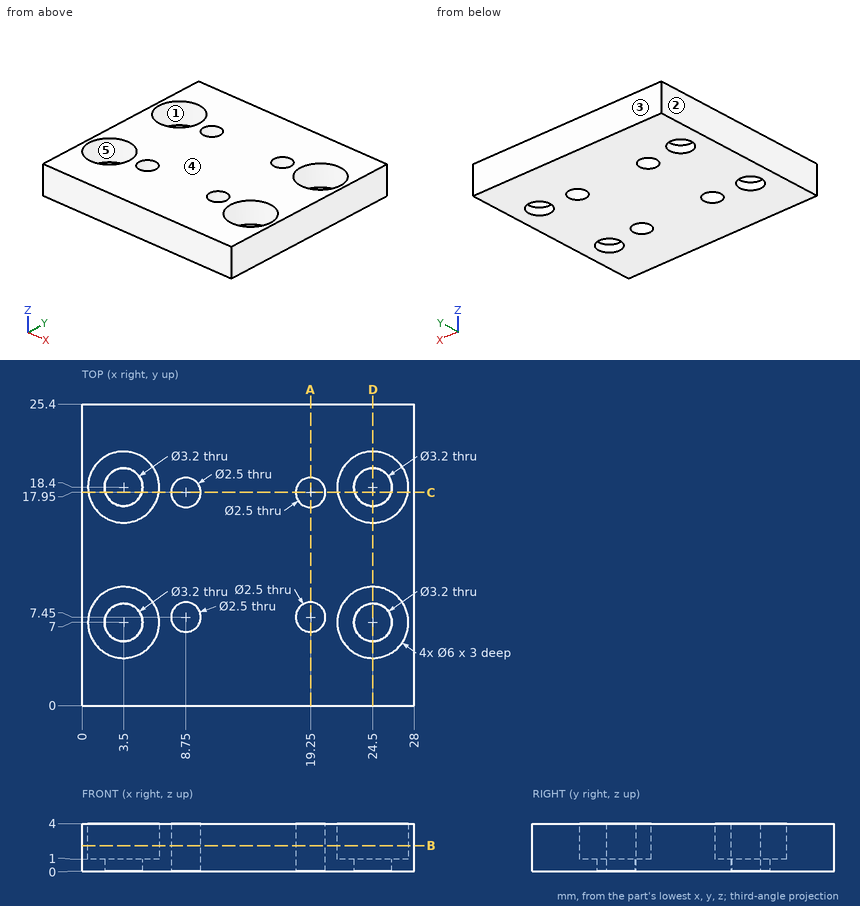
Print and shaded views of the part. All mm, measured from the part's lowest x, y and z. A direction names the side the tool comes from. Coordinates: 2 decimals unless noted, no trailing zeros. Write each loop counter-clockwise with the first axis right and the second up, starting at its lowest first coordinate (ties: lowest second). Pieces come first, ordered by that corner, then holes. Notation, with made-up numbers: M 49.5,74.5 L 88.5,74.5 A23 cw 88.5,90.5 Z; hole C 14.5,16 d1. An arc over 180 degrees is marked long. Return JSON: item names as keys, results as strings.
1. Probe L1, parallel to X at y = 18.4, z = 0.2; L2, parallel to X at y = 9, z = 1.9; L3, parallel to Y at x = 8.5, z = 2.35. List the from-to ranges inside material, lowest first.
Determined:
{"L1": "0 to 1.9, 5.1 to 7.58, 9.92 to 18.08, 20.42 to 22.9, 26.1 to 28", "L2": "0 to 1.26, 5.74 to 22.26, 26.74 to 28", "L3": "0 to 6.23, 8.67 to 16.73, 19.17 to 25.4"}
2. 3-axis set-ups, long thin cutter, end or side, ignore diameter. For the marked faces 4 and 5: which of +Z, -Z, +X, -X, +Y, -Y reach the whole face in a straight line?
Determined:
{"face 4": "+Z, +X, -X, +Y, -Y", "face 5": "+Z"}
3. Saw through at D-D, the plane x = 24.5. Write the cut outline in (y, z), then the cut area to 3 significant figures.
Determined:
{"outline": "M 0,0 L 5.4,0 L 5.4,1 L 4,1 L 4,4 L 0,4 Z; M 8.6,0 L 16.8,0 L 16.8,1 L 15.4,1 L 15.4,4 L 10,4 L 10,1 L 8.6,1 Z; M 20,0 L 25.4,0 L 25.4,4 L 21.4,4 L 21.4,1 L 20,1 Z", "area": "59.2 mm²"}
4. Saw through at A-A, the plane x = 19.25. Write the cut outline in (y, z).
Determined:
{"outline": "M 0,0 L 6.2,0 L 6.2,4 L 0,4 Z; M 8.7,0 L 16.7,0 L 16.7,4 L 8.7,4 Z; M 19.2,0 L 25.4,0 L 25.4,4 L 19.2,4 Z"}
5. Saw through at C-C, the plane y = 17.95. Write the cut outline in (x, z).
Determined:
{"outline": "M 0,0 L 1.96,0 L 1.96,1 L 0.53,1 L 0.53,4 L 0,4 Z; M 5.04,0 L 7.5,0 L 7.5,4 L 6.47,4 L 6.47,1 L 5.04,1 Z; M 10,0 L 18,0 L 18,4 L 10,4 Z; M 20.5,0 L 22.96,0 L 22.96,1 L 21.53,1 L 21.53,4 L 20.5,4 Z; M 26.04,0 L 28,0 L 28,4 L 27.47,4 L 27.47,1 L 26.04,1 Z"}
6. Pull direction Y, two halves, no side cores. Call the marked faces 1, 2 and 3: pulls with the +Y half, pulls with the -Y half, needs draft (parallel to the pull), parting line crosses it, or undercut.
Determined:
{"face 1": "undercut", "face 2": "needs draft", "face 3": "pulls with the +Y half"}
7. Saw through at B-B, the plane z = 2.15. Count the separate pieces of the cut face and the enclosed holes in it, then the cut area to 3 significant figures.
Determined:
{"separate pieces": "1", "enclosed holes": "8", "area": "578 mm²"}
8. Flat gauge pins, fed straight in: pin 1 Ø3 at (x, y) = (20.5, 7.5) entering from -Z; pin 2 Ø1.8 at (x, y) = (25.5, 7.5) entering from +Z. Where does each tip first touch, or does it go through?
Determined:
{"pin 1": "z = 0", "pin 2": "z = 1"}
